```python
from build123d import *

# Parameters (mm, degrees)
F0_R     = 3.175
F1_DEPTH = 3.175
F2_R     = 1.5875
F3_DEPTH = 34.925


with BuildPart() as f1:
    # F0 (on Top) → F1 (new body)
    with BuildSketch(Plane.XY):
        Circle(F0_R)
        Polygon((-1.833087, 0), (-0.916544, 1.5875), (0.916544, 1.5875), (1.833087, 0), (0.916544, -1.5875), (-0.916544, -1.5875), align=None, mode=Mode.SUBTRACT)
    extrude(amount=F1_DEPTH)

    # F2 (on Top) → F3 (cut)
    with BuildSketch(Plane.XY):
        Circle(F2_R)
    extrude(amount=-F3_DEPTH, mode=Mode.SUBTRACT)


solid = f1.part
```
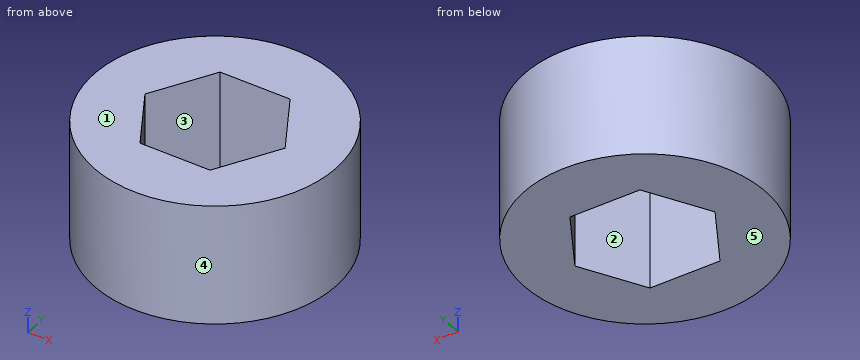
The listing builds one solid part. Answer for the finished solid, in the listing's coordinates (mm). Face numbers are marked on the shaded views. A direction names the side the tool comes from. Coordinates: 2 decimals unless noted, no trailing zeros. Loops run counter-clockwise (first coordinate to the right, second up) from the corner with the lowest first, then second, coordinate; pieces in that order, holes last. Notation, with made-up numbers: (29.5, 28.25) - (67.5, 28.25) arc R21 cw to (67.5, 64.25) - close; hole circle Ø9 at (-39, 46). An arc over 180 degrees is marked (long way). Use a Markdown table: item, result. Add a question column.
1) Find the intervals of material crossed by line 1 (Y direction, x = 0, z = 2.8) (1 decimal); line 2 (X direction, y = 0.75, z = 1.85); line 3 (X direction, y = -1.25, z = 0.95), in increasing order.
2) For the marked faces 1 and 2, determine the directions among +Z, -Z, +X, -X, +Y, -Y from which every point of the face is accessible in a straight line to the end or side of a thin tool.
3) The part is cut by section B-B, the plane y = -1.25. Give the vertices of the cut face in (x, z) (3 decimals), and give its area (3 significant figures).
4) The mould has two halves that part along Y. Classify the marked faces 3, 4 and 5: released by +Y, released by -Y, zero draft, split by the parting line, or undercut.
5) The part is cut by section D-D, the plane y = -2.5. Give the vertices of the cut face in (x, z) (3 decimals), and give its area (3 significant figures).
6) The part is cut by section A-A, the plane x = 0. Give the vertices of the cut face in (y, z) (1 decimal), and give its area (3 significant figures).
Here are the results:
| question | item | result |
|---|---|---|
| 1 | line 1 | y = -3.2 to -1.6, 1.6 to 3.2 |
| 1 | line 2 | x = -3.09 to -1.4, 1.4 to 3.09 |
| 1 | line 3 | x = -2.92 to -1.11, 1.11 to 2.92 |
| 2 | face 1 | +Z, +X, -X, +Y, -Y |
| 2 | face 2 | +Z, -Z |
| 3 | outline | (-2.919, 0) - (-1.111, 0) - (-1.111, 3.175) - (-2.919, 3.175) - close; (1.111, 0) - (2.919, 0) - (2.919, 3.175) - (1.111, 3.175) - close |
| 3 | area | 11.5 mm^2 |
| 4 | face 3 | undercut |
| 4 | face 4 | split by the parting line |
| 4 | face 5 | zero draft |
| 5 | outline | (-1.957, 0) - (1.957, 0) - (1.957, 3.175) - (-1.957, 3.175) - close |
| 5 | area | 12.4 mm^2 |
| 6 | outline | (-3.2, 0) - (-1.6, 0) - (-1.6, 3.2) - (-3.2, 3.2) - close; (1.6, 0) - (3.2, 0) - (3.2, 3.2) - (1.6, 3.2) - close |
| 6 | area | 10.1 mm^2 |
